The listing builds one solid part. Answer for the finished solid, in the listing's coordinates (mm). Coordinates: 2 decimals unless noted, no trailing zeros. Order: outer loops, then holes, each group sorted by start corner. A loop starts at its lowest first (then second) coordinate and runs counter-clockwise, first axis right, second up.
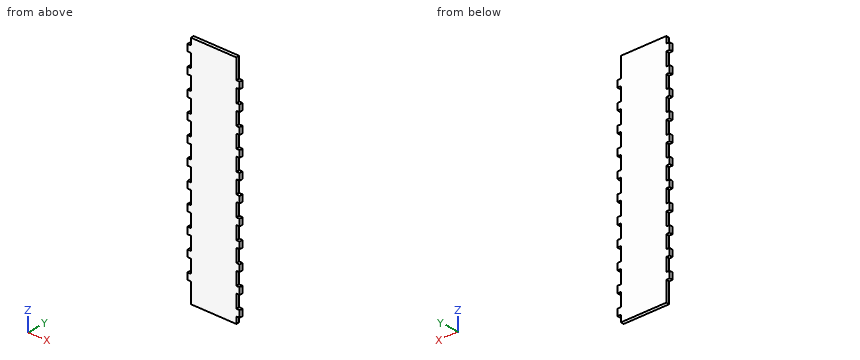
from build123d import *

# Parameters (mm, degrees)
BOSS_EXTRUDE1_DEPTH = 5


with BuildPart() as part:
    # Sketch1 → Boss-Extrude1 (new body)
    with BuildSketch(Plane(origin=(0, 0, 0), x_dir=(1, 0, 0), z_dir=(0, 1, 0))):
        Polygon((-238.169070324, -88.755561118), (-238.169070324, -78.755561118), (-233.169070324, -78.755561118), (-233.169070324, -58.755561118), (-238.169070324, -58.755561118), (-238.169070324, -48.755561118), (-233.169070324, -48.755561118), (-233.169070324, -28.755561118), (-238.169070324, -28.755561118), (-238.169070324, -18.755561118), (-233.169070324, -18.755561118), (-233.169070324, 1.244438882), (-238.169070324, 1.244438882), (-238.169070324, 11.244438882), (-233.169070324, 11.244438882), (-233.169070324, 31.244438882), (-238.169070324, 31.244438882), (-238.169070324, 41.244438882), (-233.169070324, 41.244438882), (-233.169070324, 61.244438882), (-238.169070324, 61.244438882), (-238.169070324, 71.244438882), (-233.169070324, 71.244438882), (-233.169070324, 91.244438882), (-238.169070324, 91.244438882), (-238.169070324, 101.244438882), (-233.169070324, 101.244438882), (-233.169070324, 121.244438882), (-238.169070324, 121.244438882), (-238.169070324, 131.244438882), (-233.169070324, 131.244438882), (-233.169070324, 151.244438882), (-238.169070324, 151.244438882), (-238.169070324, 161.244438882), (-233.169070324, 161.244438882), (-233.169070324, 181.244438882), (-238.169070324, 181.244438882), (-238.169070324, 191.244438882), (-233.169070324, 191.244438882), (-233.169070324, 211.244438882), (-233.169070324, 221.244438882), (-163.169070324, 221.244438882), (-163.169070324, 211.244438882), (-158.169070324, 211.244438882), (-158.169070324, 201.244438882), (-163.169070324, 201.244438882), (-163.169070324, 181.244438882), (-158.169070324, 181.244438882), (-158.169070324, 171.244438882), (-163.169070324, 171.244438882), (-163.169070324, 151.244438882), (-158.169070324, 151.244438882), (-158.169070324, 141.244438882), (-163.169070324, 141.244438882), (-163.169070324, 121.244438882), (-158.169070324, 121.244438882), (-158.169070324, 111.244438882), (-163.169070324, 111.244438882), (-163.169070324, 91.244438882), (-158.169070324, 91.244438882), (-158.169070324, 81.244438882), (-163.169070324, 81.244438882), (-163.169070324, 61.244438882), (-158.169070324, 61.244438882), (-158.169070324, 51.244438882), (-163.169070324, 51.244438882), (-163.169070324, 31.244438882), (-158.169070324, 31.244438882), (-158.169070324, 21.244438882), (-163.169070324, 21.244438882), (-163.169070324, 1.244438882), (-158.169070324, 1.244438882), (-158.169070324, -8.755561118), (-163.169070324, -8.755561118), (-163.169070324, -28.755561118), (-158.169070324, -28.755561118), (-158.169070324, -38.755561118), (-163.169070324, -38.755561118), (-163.169070324, -58.755561118), (-158.169070324, -58.755561118), (-158.169070324, -68.755561118), (-163.169070324, -68.755561118), (-163.169070324, -88.755561118), (-158.169070324, -88.755561118), (-158.169070324, -98.755561118), (-163.169070324, -98.755561118), (-163.169070324, -118.755561118), (-163.169070324, -128.755561118), (-233.169070324, -128.755561118), (-233.169070324, -118.755561118), (-238.169070324, -118.755561118), (-238.169070324, -108.755561118), (-233.169070324, -108.755561118), (-233.169070324, -88.755561118), align=None)
    extrude(amount=BOSS_EXTRUDE1_DEPTH)


solid = part.part
(1) Find section A-A on z = -35. Determine the outline of the cut face in (x, y).
(2) Given pin 1 Ø2.5 at (x, y) = (-160, 2) entering from -Z; pin 2 Ø2.5 at (x, y) = (-235, 3) entering from -Z; pin 3 Ø2.5 at (y, z) = (3.5, -170) entering from -X, each flat-ended and moving along its own axis, determine where each tip first touches the part or whether it passes through.
(3) Find the intervals of material crossed by probe 1 along X at (y, z) = (4.35, -170); probe 2 along X at (y, z) = (2.75, -29.5), in increasing order.
Resolved:
1. outline: (-238.17, 0) - (-163.17, 0) - (-163.17, 5) - (-238.17, 5) - close
2. pin 1: stops at z = -211.24
2. pin 2: stops at z = -191.24
2. pin 3: stops at x = -233.17
3. probe 1: x = -233.17 to -163.17
3. probe 2: x = -233.17 to -158.17
